Geometry check sheet. Reference: the model listing, model coordinates, mm. Face numbers are marked on the shaded views. A direction names the side the tool comes from. Round coordinates to 2 decimals unless told otherwise and drop trailing zeros. Write each loop counter-clockwise with the first axis right and the second up, starting at its lowest first coordinate (ties: lowest second). Pieces come first, ordered by that corner, then holes. Notation, with made-up numbers: (26, -14) - (75, -14) arc R13 cw to (75, 9) - close; hole circle Ø2 at (17, 44.5). An arc over 180 degrees is marked (long way). Return JSON: item names as keys, results as strings.
```python
from build123d import *

# Parameters (mm, degrees)
BOSS_EXTRUDE1_DEPTH = 80
BOSS_EXTRUDE2_DEPTH = 2.5
SKETCH4_W           = 8.75
SKETCH4_H           = 75
SKETCH5_R           = 2.05
CUT_EXTRUDE1_DEPTH  = 4.1


with BuildPart() as part:
    # Sketch1 → Boss-Extrude1 (new body)
    with BuildSketch(Plane.XY):
        with BuildLine():
            Line((-70, 0), (70, 0))
            Line((70, 0), (70, 15))
            Line((70, 15), (39.686269666, 15))
            ThreePointArc((39.686269666, 15), (53.810362803, 33.458619949), (59.859752756, 55.9))
            Line((59.859752756, 55.9), (75, 55.9))
            Line((75, 55.9), (75, 60))
            Line((75, 60), (48.75, 60))
            ThreePointArc((48.75, 60), (0, 11.25), (-48.75, 60))
            Line((-48.75, 60), (-75, 60))
            Line((-75, 60), (-75, 55.9))
            Line((-75, 55.9), (-59.859752756, 55.9))
            ThreePointArc((-59.859752756, 55.9), (-53.810362803, 33.458619949), (-39.686269666, 15))
            Line((-39.686269666, 15), (-70, 15))
            Line((-70, 15), (-70, 0))
        make_face()
    extrude(amount=BOSS_EXTRUDE1_DEPTH)

    # Sketch3 → Boss-Extrude2 (add)
    with BuildSketch(Plane(origin=(0, 0, 0), x_dir=(-1, 0, 0), z_dir=(0, 0, -1))):
        with BuildLine():
            ThreePointArc((-15, 60), (0, 45), (15, 60))
            Line((15, 60), (48.75, 60))
            ThreePointArc((48.75, 60), (0, 11.25), (-48.75, 60))
            Line((-48.75, 60), (-15, 60))
        make_face()
    extrude(amount=-BOSS_EXTRUDE2_DEPTH)

    # Sketch4 → Cut-Revolve1 (revolve, cut)
    with BuildSketch(Plane(origin=(0, 60, 0), x_dir=(1, 0, 0), z_dir=(0, 1, 0))):
        with Locations((-53.125, -40)):
            Rectangle(SKETCH4_W, SKETCH4_H)
    revolve(axis=Axis((0, 60, 0), (0, 0, 1)), mode=Mode.SUBTRACT)

    # Sketch5 → Cut-Extrude1 (cut)
    with BuildSketch(Plane(origin=(0, 60, 0), x_dir=(1, 0, 0), z_dir=(0, 1, 0))):
        with Locations(Location((67.5, -70, 0), (0, 0, 270))):
            Circle(SKETCH5_R)
        with Locations(Location((67.5, -50, 0), (0, 0, 270))):
            Circle(SKETCH5_R)
        with Locations(Location((67.5, -30, 0), (0, 0, 270))):
            Circle(SKETCH5_R)
        with Locations(Location((67.5, -10, 0), (0, 0, 270))):
            Circle(SKETCH5_R)
        with Locations(Location((-67.5, -10, 0), (0, 0, 180))):
            Circle(SKETCH5_R)
        with Locations(Location((-67.5, -30, 0), (0, 0, 180))):
            Circle(SKETCH5_R)
        with Locations(Location((-67.5, -50, 0), (0, 0, 180))):
            Circle(SKETCH5_R)
        with Locations(Location((-67.5, -70, 0), (0, 0, 180))):
            Circle(SKETCH5_R)
    extrude(amount=-CUT_EXTRUDE1_DEPTH, mode=Mode.SUBTRACT)


solid = part.part
```
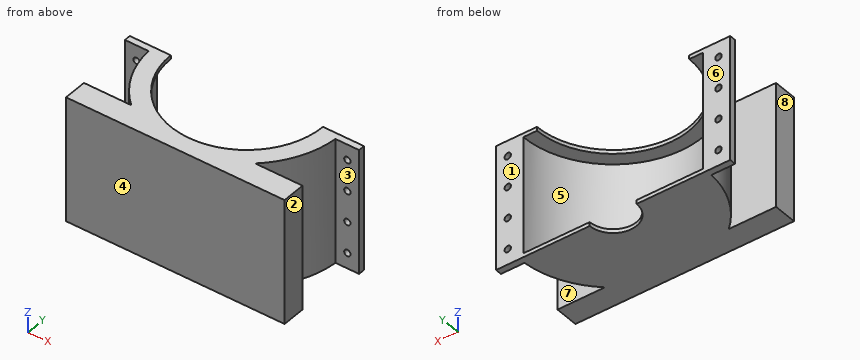
(1) Material ranges on line 1 along Y through (x, z) = (-62.5, 69); line 2 along Z through (x, y) = (-67, 56); line 3 along Z through (x, y) = (-29, 45.5), recorded low to high. Write a range as [from, to].
Response values:
{"line 1": "y = [0, 15], [55.9, 60]", "line 2": "z = [0, 8.01], [11.99, 28.01], [31.99, 48.01], [51.99, 68.01], [71.99, 80]", "line 3": "z = [0, 2.5]"}
(2) Section check D-D, the plane x = 0. Enter the section's corners in (y, z).
Response values:
{"outline": "(0, 0) - (45, 0) - (45, 2.5) - (2.5, 2.5) - (2.5, 77.5) - (11.25, 77.5) - (11.25, 80) - (0, 80) - close"}
(3) Section check A-A, the plane x = 67.5. Enter the section's corners in (y, z), plus the area to 3 significant figures.
Response values:
{"outline": "(0, 0) - (15, 0) - (15, 80) - (0, 80) - close; (55.9, 0) - (60, 0) - (60, 7.95) - (55.9, 7.95) - close; (55.9, 12.05) - (60, 12.05) - (60, 27.95) - (55.9, 27.95) - close; (55.9, 32.05) - (60, 32.05) - (60, 47.95) - (55.9, 47.95) - close; (55.9, 52.05) - (60, 52.05) - (60, 67.95) - (55.9, 67.95) - close; (55.9, 72.05) - (60, 72.05) - (60, 80) - (55.9, 80) - close", "area": "1,460 mm^2"}
(4) Access from +Z, -Z, +X, -X, +Y, -Y to the whole of each face (thin tool, end or side, straight path). Record for the marked faces 1, 2, 3, 4 and 5.
Response values:
{"face 1": "+Z, -Z, +X, -X, +Y", "face 2": "+Z, -Z, +X, -Y", "face 3": "+Z, -Z, +X", "face 4": "+Z, -Z, +X, -X, -Y", "face 5": "+Y"}
(5) Section check B-B, the plane y = 46.5. Enter the section's corners in (x, z).
Response values:
{"outline": "(-58.46, 0) - (-6.54, 0) - (-6.54, 2.5) - (-55.89, 2.5) - (-55.89, 77.5) - (-46.84, 77.5) - (-46.84, 80) - (-58.46, 80) - close; (6.54, 0) - (58.46, 0) - (58.46, 80) - (46.84, 80) - (46.84, 77.5) - (55.89, 77.5) - (55.89, 2.5) - (6.54, 2.5) - close"}
(6) Gauge pin test, flat ends, axial feed: pin 1 (7.5 mm diameter, centred on y = 11, z = 54.5, fed in from -X); pin 2 (16.5 mm diameter, centred on y = 10.5, z = 24.5, fed in from +X); pin 3 (3.5 mm diameter, centred on x = 67.5, z = 70, fed in from +Y). Record the tip position at first contact, or that the pin passes through.
Response values:
{"pin 1": "stops at x = -70", "pin 2": "stops at x = 70", "pin 3": "stops at y = 15"}
(7) Section check C-C, the plane z = 50. Enter the section's corners in (x, y).
Response values:
{"outline": "(-75, 55.9) - (-69.55, 55.9) - (-69.55, 60) - (-75, 60) - close; (-70, 0) - (70, 0) - (70, 15) - (39.69, 15) arc R60 ccw to (59.86, 55.9) - (65.45, 55.9) - (65.45, 60) - (57.5, 60) arc R57.5 cw to (-57.5, 60) - (-65.45, 60) - (-65.45, 55.9) - (-59.86, 55.9) arc R60 ccw to (-39.69, 15) - (-70, 15) - close; (69.55, 55.9) - (75, 55.9) - (75, 60) - (69.55, 60) - close"}
(8) Release check for a two-part mould opening along Y. For the marked faces 6, 7 and 8 record: pulls with the +Y half, pulls with the -Y half, needs draft (parallel to the pull), parting line crosses it, or undercut.
Response values:
{"face 6": "pulls with the +Y half", "face 7": "undercut", "face 8": "needs draft"}
